The drawing under review shows one solid part. Ordinate dimensions are in mm from its lowest x, y, z. A direction names the side the tool comes from. Give positions to 0.01 mm unless a question says otherwise; leave off trailing zeros. Loops run counter-clockwise (first coordinate to the right, second up) from the corner with the lowest first, then second, coordinate; pieces in that order, holes last. Notation, with made-up numbers: M 10,42 L 57,42 A17 ccw 57,71 Z; hole C 58.25,17 d8. An arc over 180 degrees is marked long. One line per item, written item: value. Start each with the question number.
Q1. To check wall thickness, follow line 1 along X through (y, z) = (20.5, 114); line 2 along Y through (x, z) = (52, 60); line 3 along Y through (x, z) = (9, 62). State the ranges of each line that lie inside material, in increasing order. Write a range as from..to.
Q2. For pin 1 (5.5 mm diameter, centred on x = 97.43, z = 59.38, fed in from -Y); pin 2 (4 mm diameter, centred on x = 42.5, z = 87.5, fed in from +Y) (1 decimal); pin 3 (3 mm diameter, centred on x = 32, z = 71.5, fed in from -Y) (1 decimal), all flat-tipped, find the tip position at first contact; note any pin that passes through.
Q3. For the marked faces 1 and 2, list the 3-axis set-ups (+Z, -Z, +X, -X, +Y, -Y) from which the entire face can be reached by the end or side of a thin tool; tool diameter is ignored.
Q4. We need section A-A on y = 64.5. Write out the cut boundary in (x, z) (1 decimal), plus the area to 3 significant figures.
Q5. We need section D-D on z = 109. Write out the cut boundary in (x, y), plus the area to 3 significant figures.
Q6. We need section B-B on z = 38. Write out the cut boundary in (x, y).
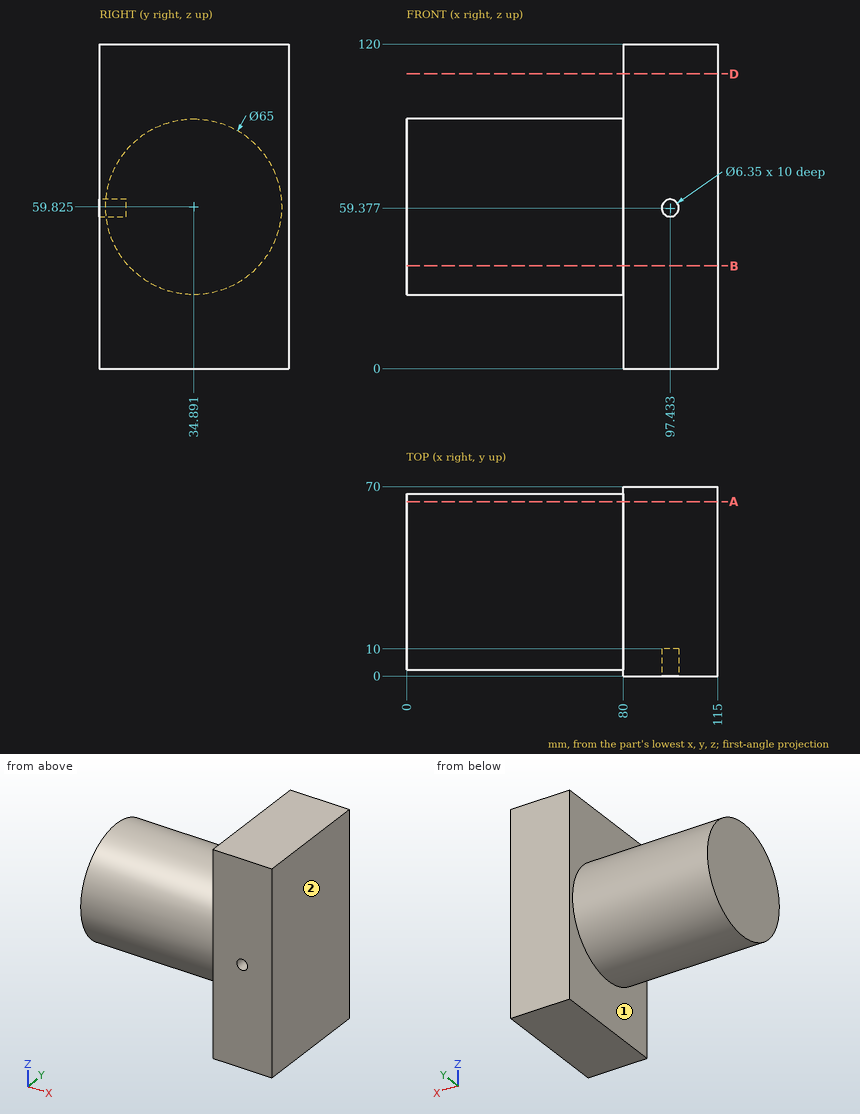
Solved:
1. line 1: 80..115
1. line 2: 2.39..67.39
1. line 3: 2.46..67.32
2. pin 1: y = 10
2. pin 2: y = 54.8
2. pin 3: y = 4
3. face 1: -X
3. face 2: +Z, -Z, +X, +Y, -Y
4. outline: M 0,46.4 L 80,46.4 L 80,0 L 115,0 L 115,120 L 80,120 L 80,73.2 L 0,73.2 Z
4. area: 6,340 mm2
5. outline: M 80,0 L 115,0 L 115,70 L 80,70 Z
5. area: 2,450 mm2
6. outline: M 0,10.81 L 80,10.81 L 80,0 L 115,0 L 115,70 L 80,70 L 80,58.97 L 0,58.97 Z
